from build123d import *

# Parameters (mm, degrees)
SKETCH_1_W             = 16.26
SKETCH_1_H             = 21.6
EXTRUDE_1_DEPTH        = 13.84
SKETCH_2_R             = 1.5
EXTRUDE_2_DEPTH        = 3
FILLET_1_R             = 0.5
SKETCH_3_W             = 0.5
SKETCH_3_H             = 1.5
EXTRUDE_3_DEPTH        = 3
FILLET_2_R             = 0.5
SKETCH_4_R             = 0.4
EXTRUDE_4_DEPTH        = 3
SKETCH_5_R             = 0.35
EXTRUDE_5_DEPTH        = 3
PATTERN_LINEAR_1_COUNT = 4
PATTERN_LINEAR_1_PITCH = 2.54
CHAMFER_1_SIZE         = 0.2
CUT_EXTRUDE_1_DEPTH    = 13
SKETCH_7_W             = 2.3
SKETCH_7_H             = 1.3
EXTRUDE_6_DEPTH        = 0.2
SKETCH_8_W             = 2.3
SKETCH_8_H             = 1.3
EXTRUDE_7_DEPTH        = 0.2


with BuildPart() as part:
    # Эскиз1 → Бобышка-Вытянуть1 (new body)
    with BuildSketch(Plane(origin=(0, 0, 0), x_dir=(1, 0, 0), z_dir=(0, 1, 0))):
        Rectangle(SKETCH_1_W, SKETCH_1_H)
    extrude(amount=EXTRUDE_1_DEPTH)

    # Эскиз2 → Бобышка-Вытянуть2 (add)
    with BuildSketch(Plane(origin=(0, 0, 0), x_dir=(1, 0, 0), z_dir=(0, 1, 0))):
        with Locations(Location((5.72, 0.1, 0), (0, 0, 270))):
            Circle(SKETCH_2_R)
        with Locations(Location((-5.72, 0.1, 0), (0, 0, 270))):
            Circle(SKETCH_2_R)
    extrude(amount=-EXTRUDE_2_DEPTH)

    # Скругление1
    fillet_1_edges = [part.edges().sort_by_distance(p)[0] for p in [
        (5.72, -3, -1.6),
        (-5.72, -3, -1.6),
    ]]
    fillet(fillet_1_edges, radius=FILLET_1_R)

    # Эскиз3 → Бобышка-Вытянуть3 (add)
    with BuildSketch(Plane(origin=(0, 0, 0), x_dir=(1, 0, 0), z_dir=(0, 1, 0))):
        with Locations((-7.88, 3.15)):
            Rectangle(SKETCH_3_W, SKETCH_3_H)
        with Locations((7.88, 3.15)):
            Rectangle(SKETCH_3_W, SKETCH_3_H)
    extrude(amount=-EXTRUDE_3_DEPTH)

    # Скругление2
    fillet_2_edges = [part.edges().sort_by_distance(p)[0] for p in [
        (-7.88, -3, -2.4),
        (-7.88, -3, -3.9),
        (7.88, -3, -2.4),
        (7.88, -3, -3.9),
    ]]
    fillet(fillet_2_edges, radius=FILLET_2_R)

    # Эскиз4 → Бобышка-Вытянуть4 (add)
    with BuildSketch(Plane(origin=(0, 0, 0), x_dir=(1, 0, 0), z_dir=(0, 1, 0))):
        with Locations(Location((-6.63, -3.96, 0), (0, 0, 270))):
            Circle(SKETCH_4_R)
        with Locations(Location((-4.09, -3.96, 0), (0, 0, 270))):
            Circle(SKETCH_4_R)
        with Locations(Location((4.09, -3.96, 0), (0, 0, 270))):
            Circle(SKETCH_4_R)
        with Locations(Location((6.63, -3.96, 0), (0, 0, 270))):
            Circle(SKETCH_4_R)
    extrude(amount=-EXTRUDE_4_DEPTH)

    # Эскиз5 → Бобышка-Вытянуть5 (add)
    with BuildSketch(Plane(origin=(0, 0, 0), x_dir=(1, 0, 0), z_dir=(0, 1, 0))):
        with Locations(Location((-4.45, 6.46, 0), (0, 0, 270))):
            Circle(SKETCH_5_R)
        with Locations(Location((-3.18, 9, 0), (0, 0, 270))):
            Circle(SKETCH_5_R)
    extrude_5 = extrude(amount=-EXTRUDE_5_DEPTH)

    # Линейный массив1: Бобышка-Вытянуть5 ×4
    with Locations(*[(i * PATTERN_LINEAR_1_PITCH, 0, 0) for i in range(1, PATTERN_LINEAR_1_COUNT)]):
        add(extrude_5)

    # Фаска1
    chamfer_1_edges = [part.edges().sort_by_distance(p)[0] for p in [
        (-0.64, -3, -9.35),
        (1.9, -3, -9.35),
        (4.44, -3, -9.35),
        (-1.91, -3, -6.81),
        (0.63, -3, -6.81),
        (3.17, -3, -6.81),
        (-6.63, -3, 3.56),
        (-4.09, -3, 3.56),
        (4.09, -3, 3.56),
        (6.63, -3, 3.56),
        (-4.45, -3, -6.81),
        (-3.18, -3, -9.35),
    ]]
    chamfer(chamfer_1_edges, length=CHAMFER_1_SIZE)

    # Эскиз6 → Вырез-Вытянуть1 (cut)
    with BuildSketch(Plane.XY.offset(10.8)):
        Polygon((-5.8, 11.34), (5.8, 11.34), (5.8, 4.14), (3.3, 4.14), (3.3, 2.64), (1.8, 2.64), (1.8, 1.44), (-1.8, 1.44), (-1.8, 2.64), (-3.3, 2.64), (-3.3, 4.14), (-5.8, 4.14), align=None)
    extrude(amount=-CUT_EXTRUDE_1_DEPTH, mode=Mode.SUBTRACT)

    # Эскиз7 → Бобышка-Вытянуть6 (add)
    with BuildSketch(Plane.XY.offset(10.8)):
        with Locations((-4.65, 3.29)):
            Rectangle(SKETCH_7_W, SKETCH_7_H)
    extrude(amount=EXTRUDE_6_DEPTH)

    # Эскиз8 → Бобышка-Вытянуть7 (add)
    with BuildSketch(Plane.XY.offset(10.8)):
        with Locations((4.65, 3.29)):
            Rectangle(SKETCH_8_W, SKETCH_8_H)
    extrude(amount=EXTRUDE_7_DEPTH)


solid = part.part
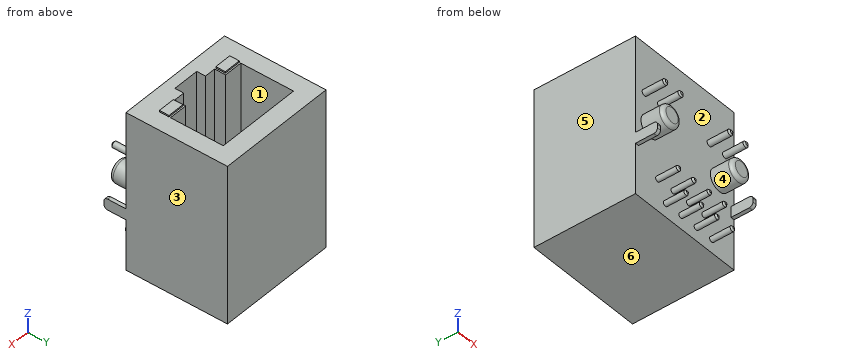
Source: CAD feature listing. Evaluate the final solid. Frame: model axes, mm. Face numbers are marked on the shaded views. A direction names the side the tool comes from. Round coordinates to 2 decimals unless told otherwise and drop trailing zeros. Loops run counter-clockwise (first coordinate to the right, second up) from the corner with the lowest first, then second, coordinate; pieces in that order, holes last. Notation, with made-up numbers: (65.25, 66) - (94.25, 66) arc R22 cw to (94.25, 90) - close; hole circle Ø11 at (21, -21.75). An arc over 180 degrees is marked (long way). Write item = value, one per line. Start each with the question number.
Item 1: Mould query, pull axis X, two halves, no side actions, for the marked faces 4, 5 and 6. Classes: released by +X, released by -X, zero draft, split by the parting line, or undercut.
Item 2: First-contact query: pin 1 Ø3 at (x, y) = (-1.5, 9) entering from +Z; pin 2 Ø0.6 at (x, y) = (8, -1) entering from +Z; pin 3 Ø3 at (x, z) = (-4, 6.5) entering from -Y. Flat tips, straight axial feed; report the tip coordinate or a pass-through.
Item 3: Reachability of the marked faces 1, 2 and 3 from +Z, -Z, +X, -X, +Y, -Y: full face, straight path, thin tool, end or side. Return the list, or none.
Item 4: Section query D-D on y = 10. Output: boundary loops of the cut face in (x, z).
Item 5: Section query B-B on y = 2. Output: boundary loops of the cut face in (x, z), plus the area to 3 significant figures.
Item 6: Section query C-C on z = -5.75. Output: boundary loops of the cut face in (x, y), plus the area to 3 significant figures.
Item 7: Section query A-A on z = 5.25. Output: boundary loops of the cut face in (x, y).
Item 8: Material intervals for line 1 (X direction, y = -2.5, z = -3.25); line 2 (Y direction, x = -1, z = 0); line 3 (X direction, y = 5.75, z = 4.75), sorted ascending.
Results list:
q1.face_4 = undercut
q1.face_5 = released by -X
q1.face_6 = zero draft
q2.pin_1 = -2.2
q2.pin_2 = -2.4
q2.pin_3 = 0
q3.face_1 = +Z
q3.face_2 = -Y
q3.face_3 = +Z, -Z, +X, +Y, -Y
q4.outline = (-8.13, -10.8) - (8.13, -10.8) - (8.13, 10.8) - (5.8, 10.8) - (5.8, -2.2) - (-5.8, -2.2) - (-5.8, 10.8) - (-8.13, 10.8) - close
q5.outline = (-8.13, -10.8) - (8.13, -10.8) - (8.13, 10.8) - (1.8, 10.8) - (1.8, -2.2) - (-1.8, -2.2) - (-1.8, 10.8) - (-8.13, 10.8) - close
q5.area = 304 mm²
q6.outline = (-8.13, 0) - (8.13, 0) - (8.13, 13.84) - (-8.13, 13.84) - close
q6.area = 225 mm²
q7.outline = (-8.13, 0) - (8.13, 0) - (8.13, 13.84) - (-8.13, 13.84) - close; hole (-5.8, 4.14) - (-3.3, 4.14) - (-3.3, 2.64) - (-1.8, 2.64) - (-1.8, 1.44) - (1.8, 1.44) - (1.8, 2.64) - (3.3, 2.64) - (3.3, 4.14) - (5.8, 4.14) - (5.8, 11.34) - (-5.8, 11.34) - close
q8.line_1 = -8.13 to -7.63, 7.63 to 8.13
q8.line_2 = 0 to 1.44, 11.34 to 13.84
q8.line_3 = -8.13 to -5.8, 5.8 to 8.13
